Could you check a few things on this model? Use its own coordinates, in mm. Face numbers are marked on the shaded views. A direction names the side the tool comes from. Round coordinates to 2 decimals unless told otherwise and drop trailing zeros. Write each loop counter-clockwise with the first axis right and the second up, starting at its lowest first coordinate (ties: lowest second). Pieces come first, ordered by that corner, then holes. Notation, with made-up numbers: (-2.5, 30.25) -> (42.5, 30.25) arc R8 cw to (42.5, 37.25) -> close; hole circle Ø2 at (7, 35.25). An arc over 180 degrees is marked (long way). Return JSON: item names as keys, results as strings.
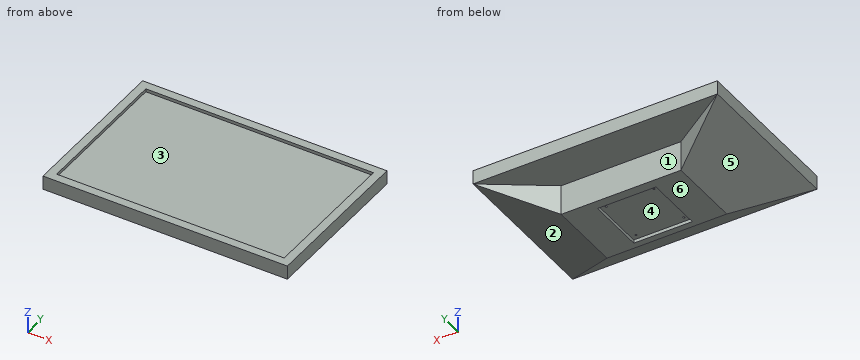
from build123d import *

# Parameters (mm, degrees)
SKETCH1_W           = 510
SKETCH1_H           = 335
BOSS_EXTRUDE1_DEPTH = 29
SKETCH2_W           = 475
SKETCH2_H           = 300
CUT_EXTRUDE1_DEPTH  = 6.5
SKETCH3_W           = 122
SKETCH3_H           = 122
BOSS_EXTRUDE2_DEPTH = 56
SKETCH4_R           = 2
CUT_EXTRUDE2_DEPTH  = 10
BOSS_EXTRUDE3_START = -56
SKETCH5_W           = 250
SKETCH5_H           = 154
SKETCH5_W_2         = 122
SKETCH5_H_2         = 122
BOSS_EXTRUDE3_DEPTH = 63
BOSS_EXTRUDE4_REACH = 360.798
BOSS_EXTRUDE5_REACH = 379.454
CUT_EXTRUDE3_DEPTH  = 63


with BuildPart() as part:
    # Sketch1 → Boss-Extrude1 (new body)
    with BuildSketch(Plane.XY):
        Rectangle(SKETCH1_W, SKETCH1_H)
    extrude(amount=-BOSS_EXTRUDE1_DEPTH)

    # Sketch2 → Cut-Extrude1 (cut)
    with BuildSketch(Plane.XY):
        Rectangle(SKETCH2_W, SKETCH2_H)
    extrude(amount=-CUT_EXTRUDE1_DEPTH, mode=Mode.SUBTRACT)

    # Sketch3 → Boss-Extrude2 (add)
    with BuildSketch(Plane(origin=(0, 0, -29), x_dir=(-1, 0, 0), z_dir=(0, 0, -1))):
        with Locations((0, 0.5)):
            Rectangle(SKETCH3_W, SKETCH3_H)
    extrude(amount=BOSS_EXTRUDE2_DEPTH)

    # Sketch4 → Cut-Extrude2 (cut)
    with BuildSketch(Plane(origin=(0, 0, -85), x_dir=(-1, 0, 0), z_dir=(0, 0, -1))):
        with Locations((-50, 50)):
            Circle(SKETCH4_R)
        with Locations((50, 50)):
            Circle(SKETCH4_R)
        with Locations((50, -50)):
            Circle(SKETCH4_R)
        with Locations((-50, -50)):
            Circle(SKETCH4_R)
    extrude(amount=-CUT_EXTRUDE2_DEPTH, mode=Mode.SUBTRACT)

    # Sketch5 → Boss-Extrude3 (add)
    with BuildSketch(Plane(origin=(0, 0, -85), x_dir=(-1, 0, 0), z_dir=(0, 0, -1)).offset(BOSS_EXTRUDE3_START)):
        with Locations((0, 3.5)):
            Rectangle(SKETCH5_W, SKETCH5_H)
        with Locations((0, 0.5)):
            Rectangle(SKETCH5_W_2, SKETCH5_H_2, mode=Mode.SUBTRACT)
    extrude(amount=BOSS_EXTRUDE3_DEPTH)

    # Sketch7 → Boss-Extrude4 (add, up to next)
    with BuildSketch(Plane(origin=(0, -65.329597813, -97.475907848), x_dir=(1, 0, 0), z_dir=(0, 0.55673786293741, 0.8306882399383573)), mode=Mode.PRIVATE) as boss_extrude4_sk1:
        Polygon((255, -122.994882164), (125, -9.835702245), (-125, -9.835702245), (-255, -122.994882164), align=None)
    boss_extrude4_tool1 = extrude(boss_extrude4_sk1.sketch, amount=BOSS_EXTRUDE4_REACH, mode=Mode.PRIVATE) - part.part
    add(boss_extrude4_tool1.solids().sort_by_distance((0, -125.859649, -56.907895))[0])

    # Sketch8 → Boss-Extrude5 (add, up to next)
    with BuildSketch(Plane(origin=(-59.87852796, 0, -123.558867219), x_dir=(0.8998964379962335, 0, -0.4361036584135601), z_dir=(0.4361036584135601, 0, 0.8998964379962335)), mode=Mode.PRIVATE) as boss_extrude5_sk1:
        Polygon((-216.826585595, 167.5), (-216.826585595, -167.5), (-72.365518175, -73.5), (-72.365518175, 80.5), align=None)
    boss_extrude5_tool1 = extrude(boss_extrude5_sk1.sketch, amount=BOSS_EXTRUDE5_REACH, mode=Mode.PRIVATE) - part.part
    boss_extrude5 = boss_extrude5_tool1.solids().sort_by_distance((-198.019768, 1.534083, -56.613497))[0]
    add(boss_extrude5)

    # Sketch9 → Cut-Extrude3 (cut)
    with BuildSketch(Plane(origin=(0, 0, -92), x_dir=(-1, 0, 0), z_dir=(0, 0, -1))):
        Polygon((0, 167.5), (255, 167.5), (125, 80.5), (0, 80.5), align=None)
    cut_extrude3 = extrude(amount=-CUT_EXTRUDE3_DEPTH, mode=Mode.SUBTRACT)

    # Mirror1: Boss-Extrude5, Cut-Extrude3 across plane
    add(boss_extrude5.mirror(Plane(origin=(0, 0, 0), x_dir=(0, 0, 1), z_dir=(1, 0, 0))))
    add(cut_extrude3.mirror(Plane(origin=(0, 0, 0), x_dir=(0, 0, 1), z_dir=(1, 0, 0))), mode=Mode.SUBTRACT)


solid = part.part
1) I want a section at B-B, the plane x = 33.5. Please give me the cut outline in (y, z).
Return value:
{"outline": "(-167.5, -29) -> (-73.5, -92) -> (-60.5, -92) -> (-60.5, -85) -> (61.5, -85) -> (61.5, -92) -> (80.5, -92) -> (80.5, -29) -> (167.5, -29) -> (167.5, 0) -> (150, 0) -> (150, -6.5) -> (-150, -6.5) -> (-150, 0) -> (-167.5, 0) -> close"}
2) For the marked faces 1, 2 and 3, which set-ups out of +Z, -Z, +X, -X, +Y, -Y let a thin tool reach every point of the face, with its end or its side?
Return value:
{"face 1": "-Z, +Y", "face 2": "-Z, +X, +Y, -Y", "face 3": "+Z"}
3) Will these pins go through, and if not, where does the flat tip stop? pin 1 Ø8 at (x, z) = (-97, -39.5) entering from +Y; pin 2 Ø4 at (x, y) = (35.5, 7) entering from +Z; pin 3 Ø12 at (y, z) = (-67, -65) entering from +X.
Return value:
{"pin 1": "y = 80.5", "pin 2": "z = -6.5", "pin 3": "x = 193.1"}
4) I want a section at C-C, the plane y = -115. Please give me the cut outline in (x, z).
Return value:
{"outline": "(-255, -29) -> (-182.39, -64.19) -> (182.39, -64.19) -> (255, -29) -> (255, 0) -> (237.5, 0) -> (237.5, -6.5) -> (-237.5, -6.5) -> (-237.5, 0) -> (-255, 0) -> close"}
5) Thinking about a two-plate mould opening in X: for the marked faces 4, 5 and 6, which applies, pulls with the +X half, pulls with the -X half, needs draft (parallel to the pull), parting line crosses it, or undercut?
Return value:
{"face 4": "undercut", "face 5": "pulls with the -X half", "face 6": "needs draft"}
6) I want a section at D-D, the plane z = -57. Please give me the cut outline in (x, y), and give its area (3 significant figures).
Return value:
{"outline": "(-197.22, -125.72) -> (197.22, -125.72) -> (197.22, 128.83) -> (125, 80.5) -> (-125, 80.5) -> (-197.22, 128.83) -> close", "area": "84,800 mm²"}
7) If I drill on probe 1 along Y at (x, z) = (50, -81); probe 2 along Y at (x, z) = (-50, -79); probe 3 along Z at (x, y) = (-114, -25), over which ranges is the centre line in solid material (lowest first)? Write a range as [from, to].
Return value:
{"probe 1": "[-89.91, -52], [-48, 48], [52, 80.5]", "probe 2": "[-92.9, -52], [-48, 48], [52, 80.5]", "probe 3": "[-92, -6.5]"}
8) I want a section at A-A, the plane x = -196.5. Please give me the cut outline in (y, z), and give its area (3 significant figures).
Return value:
{"outline": "(-167.5, -29) -> (-125.2, -57.35) -> (128.35, -57.35) -> (128.35, -29) -> (167.5, -29) -> (167.5, 0) -> (150, 0) -> (150, -6.5) -> (-150, -6.5) -> (-150, 0) -> (-167.5, 0) -> close", "area": "15,600 mm²"}
